```python
from build123d import *

# Parameters (mm, degrees)
F0_R     = 12.7
F1_DEPTH = 12.7
F4_R     = 31.75
F5_DEPTH = 3.175
F6_R     = 6.096
F7_DEPTH = 19.05
F8_DEPTH = 25.4


with BuildPart() as f1:
    # F0 (on Top) → F1 (new body)
    with BuildSketch(Plane.XY):
        Circle(F0_R)
        with BuildLine():
            ThreePointArc((8.614346, 1.798068), (8.753463, 0.903814), (8.8, 0))
            ThreePointArc((8.8, 0), (8.753463, -0.903814), (8.614346, -1.798068))
            Line((8.614346, -1.798068), (10.468267, -2.86843))
            Line((10.468267, -2.86843), (7.718267, -7.63157))
            Line((7.718267, -7.63157), (5.864346, -6.561208))
            ThreePointArc((5.864346, -6.561208), (4.4, -7.621024), (2.75, -8.359276))
            Line((2.75, -8.359276), (2.75, -10.5))
            Line((2.75, -10.5), (-2.75, -10.5))
            Line((-2.75, -10.5), (-2.75, -8.359276))
            ThreePointArc((-2.75, -8.359276), (-4.4, -7.621024), (-5.864346, -6.561208))
            Line((-5.864346, -6.561208), (-7.718267, -7.63157))
            Line((-7.718267, -7.63157), (-10.468267, -2.86843))
            Line((-10.468267, -2.86843), (-8.614346, -1.798068))
            ThreePointArc((-8.614346, -1.798068), (-8.8, 0), (-8.614346, 1.798068))
            Line((-8.614346, 1.798068), (-10.468267, 2.86843))
            Line((-10.468267, 2.86843), (-7.718267, 7.63157))
            Line((-7.718267, 7.63157), (-5.864346, 6.561208))
            ThreePointArc((-5.864346, 6.561208), (-4.4, 7.621024), (-2.75, 8.359276))
            Line((-2.75, 8.359276), (-2.75, 10.5))
            Line((-2.75, 10.5), (2.75, 10.5))
            Line((2.75, 10.5), (2.75, 8.359276))
            ThreePointArc((2.75, 8.359276), (4.4, 7.621024), (5.864346, 6.561208))
            Line((5.864346, 6.561208), (7.718267, 7.63157))
            Line((7.718267, 7.63157), (10.468267, 2.86843))
            Line((10.468267, 2.86843), (8.614346, 1.798068))
        make_face(mode=Mode.SUBTRACT)
    extrude(amount=F1_DEPTH)

    # F4 (on face) → F5 (join)
    with BuildSketch(Plane.XY.offset(12.7)):
        Circle(F4_R)
    extrude(amount=F5_DEPTH)

    # F6 (on face) → F7 (join)
    with BuildSketch(Plane.XY.offset(15.875)):
        with Locations((0, 19.05)):
            Circle(F6_R)
        with Locations((0, -19.05)):
            Circle(F6_R)
    extrude(amount=F7_DEPTH)

    # F5_face (on face) → F8 (cut)
    with BuildSketch(Plane.XY.offset(15.875)):
        with BuildLine():
            Line((5.864346, 6.561208), (7.718267, 7.63157))
            Line((7.718267, 7.63157), (10.468267, 2.86843))
            Line((10.468267, 2.86843), (8.614346, 1.798068))
            ThreePointArc((8.614346, 1.798068), (8.8, 0), (8.614346, -1.798068))
            Line((8.614346, -1.798068), (10.468267, -2.86843))
            Line((10.468267, -2.86843), (7.718267, -7.63157))
            Line((7.718267, -7.63157), (5.864346, -6.561208))
            ThreePointArc((5.864346, -6.561208), (4.4, -7.621024), (2.75, -8.359276))
            Line((2.75, -8.359276), (2.75, -10.5))
            Line((2.75, -10.5), (-2.75, -10.5))
            Line((-2.75, -10.5), (-2.75, -8.359276))
            ThreePointArc((-2.75, -8.359276), (-4.4, -7.621024), (-5.864346, -6.561208))
            Line((-5.864346, -6.561208), (-7.718267, -7.63157))
            Line((-7.718267, -7.63157), (-10.468267, -2.86843))
            Line((-10.468267, -2.86843), (-8.614346, -1.798068))
            ThreePointArc((-8.614346, -1.798068), (-8.8, 0), (-8.614346, 1.798068))
            Line((-8.614346, 1.798068), (-10.468267, 2.86843))
            Line((-10.468267, 2.86843), (-7.718267, 7.63157))
            Line((-7.718267, 7.63157), (-5.864346, 6.561208))
            ThreePointArc((-5.864346, 6.561208), (-4.4, 7.621024), (-2.75, 8.359276))
            Line((-2.75, 8.359276), (-2.75, 10.5))
            Line((-2.75, 10.5), (2.75, 10.5))
            Line((2.75, 10.5), (2.75, 8.359276))
            ThreePointArc((2.75, 8.359276), (4.4, 7.621024), (5.864346, 6.561208))
        make_face()
    extrude(amount=-F8_DEPTH, mode=Mode.SUBTRACT)


solid = f1.part
```
The listing builds one solid part. Answer for the finished solid, in the listing's coordinates (mm). A direction names the side the tool comes from. Round coordinates to 2 decimals unless told otherwise and drop trailing zeros. Loops run counter-clockwise (first coordinate to the right, second up) from the corner with the lowest first, then second, coordinate; pieces in that order, holes last. Notation, with made-up numbers: (31, -9.5) -> (53, -9.5) arc R11 ccw to (53, 9.5) -> close; hole circle Ø9 at (2, 35). An arc over 180 degrees is marked (long way). Use one line per item in the form item = value.
1. The part is cut by section D-D on y = 0. Determine the outline of the cut face in (x, z) (3 decimals).
Answer key:
outline = (-31.75, 12.7) -> (-12.7, 12.7) -> (-12.7, 0) -> (-8.8, 0) -> (-8.8, 15.875) -> (-31.75, 15.875) -> close; (8.8, 0) -> (12.7, 0) -> (12.7, 12.7) -> (31.75, 12.7) -> (31.75, 15.875) -> (8.8, 15.875) -> close
2. Flat-ended cylindrical pins translate along their axes: pin 1 Ø5 at (x, z) = (21.5, 12) entering from +Y; pin 2 Ø6 at (x, z) = (1.5, 8.5) entering from +Y; pin 3 Ø2.5 at (y, z) = (-9, 5) entering from -X. Find the tip coordinate at first contact, or state that the pin passes through.
Answer key:
pin_1 = 25.36
pin_2 = 12.7
pin_3 = -10.06
3. The part is cut by section B-B on z = 3.5. Determine the outline of the cut face in (x, y).
Answer key:
outline = circle Ø25.4 at (0, 0); hole (-10.47, -2.87) -> (-7.72, -7.63) -> (-5.86, -6.56) arc R8.8 ccw to (-2.75, -8.36) -> (-2.75, -10.5) -> (2.75, -10.5) -> (2.75, -8.36) arc R8.8 ccw to (5.86, -6.56) -> (7.72, -7.63) -> (10.47, -2.87) -> (8.61, -1.8) arc R8.8 ccw to (8.61, 1.8) -> (10.47, 2.87) -> (7.72, 7.63) -> (5.86, 6.56) arc R8.8 ccw to (2.75, 8.36) -> (2.75, 10.5) -> (-2.75, 10.5) -> (-2.75, 8.36) arc R8.8 ccw to (-5.86, 6.56) -> (-7.72, 7.63) -> (-10.47, 2.87) -> (-8.61, 1.8) arc R8.8 ccw to (-8.61, -1.8) -> close
4. The part is cut by section C-C on y = -19.05. Determine the outline of the cut face in (x, z) (3 decimals).
Answer key:
outline = (-25.4, 12.7) -> (25.4, 12.7) -> (25.4, 15.875) -> (6.096, 15.875) -> (6.096, 34.925) -> (-6.096, 34.925) -> (-6.096, 15.875) -> (-25.4, 15.875) -> close
5. A tool of negligible diameter and unlimited length cuts with its end or side. For faces 1 (the flat face through (0, -19, 34.925)), 2 (the cylindrical face through (-6.09, -18.78, 25.27)), 3 (the flat face through (-9.528, 2.326, 8.049)), from which of +Z, -Z, +X, -X, +Y, -Y can it reach the whole face along a straight path? Write none if from no direction.
Answer key:
face_1 = +Z, +X, -X, +Y, -Y
face_2 = +Z
face_3 = +Z, -Z
6. For a pull along X with two mould halves and no side action, classify faces 4 (the flat face through (5, 8, 0)), 5 (the cylindrical face through (-2.75, -12.4, 6.26)), 6 (the flat face through (0, -10.5, 8)) as released by +X, released by -X, zero draft, split by the parting line, or undercut.
Answer key:
face_4 = zero draft
face_5 = split by the parting line
face_6 = undercut
7. The part is cut by section A-A on x = 0. Determine the outline of the cut face in (y, z) (3 decimals).
Answer key:
outline = (-31.75, 12.7) -> (-12.7, 12.7) -> (-12.7, 0) -> (-10.5, 0) -> (-10.5, 15.875) -> (-12.954, 15.875) -> (-12.954, 34.925) -> (-25.146, 34.925) -> (-25.146, 15.875) -> (-31.75, 15.875) -> close; (10.5, 0) -> (12.7, 0) -> (12.7, 12.7) -> (31.75, 12.7) -> (31.75, 15.875) -> (25.146, 15.875) -> (25.146, 34.925) -> (12.954, 34.925) -> (12.954, 15.875) -> (10.5, 15.875) -> close
8. Find the intervals of material crossed by probe 1 along Z at (x, y) = (9, 8) (3 decimals); probe 2 along Z at (x, y) = (-5, -12) (3 decimals); probe 3 along X at (y, z) = (8, 10), in increasing order. Write a range as [from, to].
Answer key:
probe_1 = [0, 15.875]
probe_2 = [12.7, 15.875]
probe_3 = [-9.86, -3.67], [3.67, 9.86]
